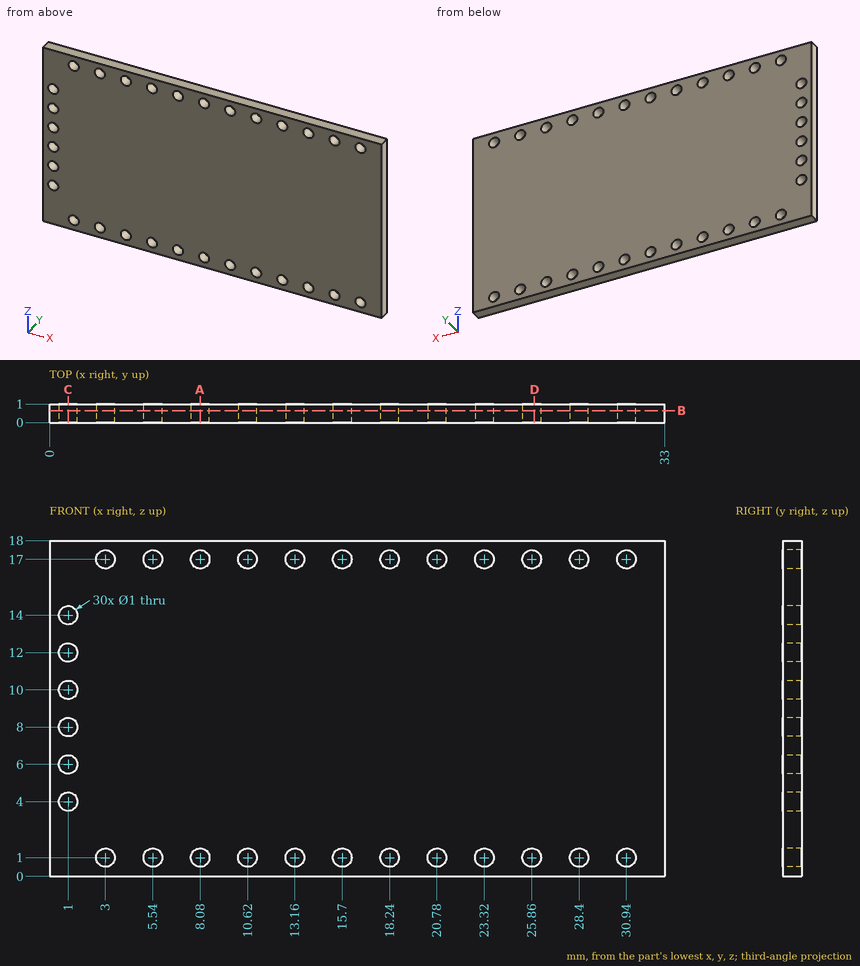
Source: three-view drawing plus pictorial views. Frame: mm from the lowest corner of the part. Round coordinates to 2 decimals unless told otherwise and drop trailing zeros. Loops run counter-clockwise (first coordinate to the right, second up) from the corner with the lowest first, then second, coordinate; pieces in that order, holes last.
Q1. Section D-D on x = 26. Return loops of the section in (y, z), plus the area to 3 significant figures.
Q2. Section C-C on x = 1. Return loops of the section in (y, z), plus the area to 3 significant figures.
Q3. Section A-A on x = 8.08. Return loops of the section in (y, z).
Q4. Material intervals for L1, parallel to Z at x = 13.16, y = 0.25; L2, parallel to X at y = 0.8, z = 4; L3, parallel to Z at x = 23, y = 0.9, sorted ascending.
Q5. Section B-B on y = 0.65. State how many separate pieces and enclosed holes the cut face has, plus the area to 3 significant figures.
Evaluation:
1. outline: (0, 0) - (1, 0) - (1, 0.52) - (0, 0.52) - close; (0, 1.48) - (1, 1.48) - (1, 16.52) - (0, 16.52) - close; (0, 17.48) - (1, 17.48) - (1, 18) - (0, 18) - close
1. area: 16.1 mm2
2. outline: (0, 0) - (1, 0) - (1, 3.5) - (0, 3.5) - close; (0, 4.5) - (1, 4.5) - (1, 5.5) - (0, 5.5) - close; (0, 6.5) - (1, 6.5) - (1, 7.5) - (0, 7.5) - close; (0, 8.5) - (1, 8.5) - (1, 9.5) - (0, 9.5) - close; (0, 10.5) - (1, 10.5) - (1, 11.5) - (0, 11.5) - close; (0, 12.5) - (1, 12.5) - (1, 13.5) - (0, 13.5) - close; (0, 14.5) - (1, 14.5) - (1, 18) - (0, 18) - close
2. area: 12.0 mm2
3. outline: (0, 0) - (1, 0) - (1, 0.5) - (0, 0.5) - close; (0, 1.5) - (1, 1.5) - (1, 16.5) - (0, 16.5) - close; (0, 17.5) - (1, 17.5) - (1, 18) - (0, 18) - close
4. L1: z = 0 to 0.5, 1.5 to 16.5, 17.5 to 18
4. L2: x = 0 to 0.5, 1.5 to 33
4. L3: z = 0 to 0.62, 1.38 to 16.62, 17.38 to 18
5. separate pieces: 1
5. enclosed holes: 30
5. area: 570 mm2
